The drawing under review shows one solid part. Ordinate dimensions are in mm from its lowest x, y, z. Give positions to 0.01 mm unless a question says otherwise; leave off trailing zeros. Write each loop counter-clockwise with the first axis right and the second up, starting at its lowest first coordinate (ties: lowest second). Pieces come first, ordered by that corner, then holes. Notation, with made-up numbers: (58, 40) - (82, 40) arc R19 ccw to (82, 66) - close; hole circle Ø10 at (77, -6.5). An arc over 180 degrees is marked (long way). Write item = value, one per line.
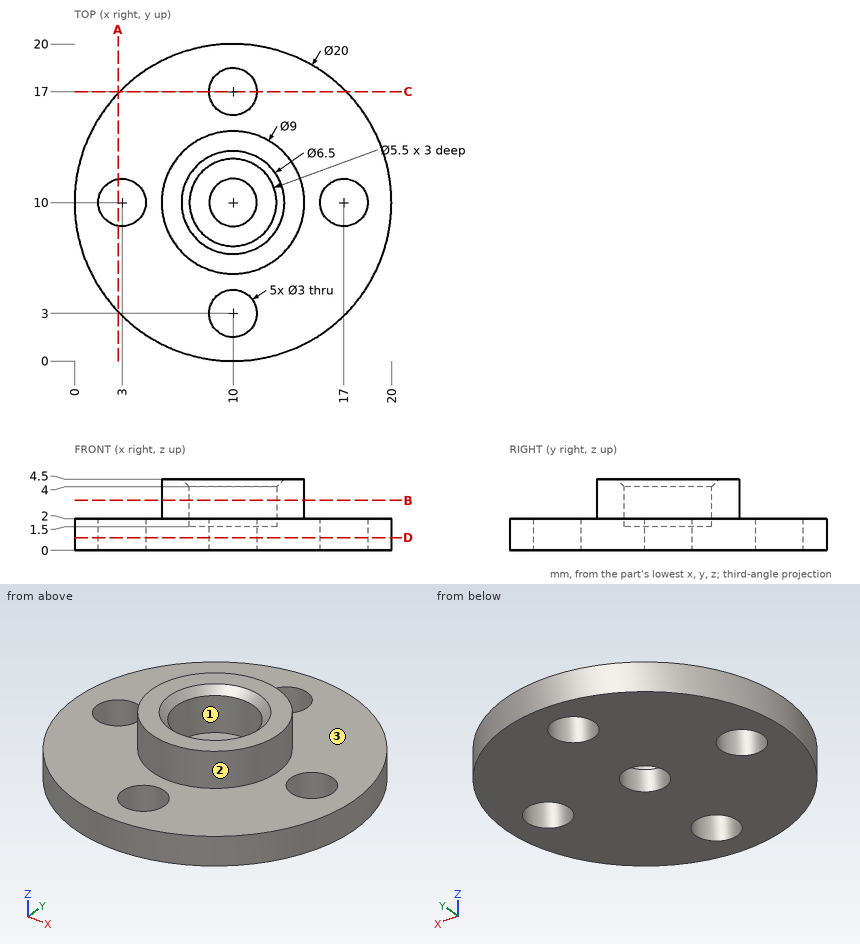
1. Take a section at D-D on z = 0.8. Give the boundary of the cut face in (x, y), and give its area (3 significant figures).
Findings below:
outline = circle Ø20 at (10, 10); hole circle Ø3 at (3, 10); hole circle Ø3 at (10, 3); hole circle Ø3 at (10, 10); hole circle Ø3 at (10, 17); hole circle Ø3 at (17, 10)
area = 279 mm²
2. Draft analysis for pull direction Y (two halves, no side actions). For the marked faces 1, 2 and 3, state which applies: +Y half, -Y half, draft (parallel to the pull), parting line (faces both ways), or undercut.
Findings below:
face_1 = undercut
face_2 = parting line
face_3 = draft
3. For line 1 (Y direction, x = 10, z = 1.25); line 2 (Z direction, x = 15.5, y = 17.75); line 3 (Y direction, x = 3, z = 0.7), list the stretches that pass through material, from the lowest coordinate up. Write a range as from..to.
Findings below:
line_1 = 0..1.5, 4.5..8.5, 11.5..15.5, 18.5..20
line_2 = 0..2
line_3 = 2.86..8.5, 11.5..17.14
4. Take a section at A-A on x = 2.75. Give the boundary of the cut face in (y, z).
Findings below:
outline = (3.11, 0) - (8.52, 0) - (8.52, 2) - (3.11, 2) - close; (11.48, 0) - (16.89, 0) - (16.89, 2) - (11.48, 2) - close
5. Insertion check: P1, Ø3.5, axis at x = 10, y = 3, coming from the +Z side; P2, Ø2, axis at y = 14, z = 0.5, coming from the +X side; P3, Ø1.6, axis at x = 9.5, y = 9, coming from the +Z side. Each pin has a flat end and moves straight along its axis. Give the tip position at first contact, or say it passes through.
Findings below:
P1 = 2
P2 = 19.54
P3 = 1.5
6. Take a section at C-C on y = 17. Give the boundary of the cut face in (x, z).
Findings below:
outline = (2.86, 0) - (8.5, 0) - (8.5, 2) - (2.86, 2) - close; (11.5, 0) - (17.14, 0) - (17.14, 2) - (11.5, 2) - close
7. Take a section at B-B on z = 3.15. Give the boundary of the cut face in (x, y), and give its area (3 significant figures).
Findings below:
outline = circle Ø9 at (10, 10); hole circle Ø5.5 at (10, 10)
area = 39.9 mm²
